Input: dimensioned drawing with shaded views. Units: mm. Origin: part minimum x, y, z. Coordinates: 2 decimals unless noted, no trailing zeros. Order: outer loops, then holes, each group sorted by start corner. A loop starts at its lowest first (then second) coordinate and runs counter-clockwise, first axis right, second up. Notation, with made-up numbers: (69.25, 20.25) -> (85.25, 20.25) arc R29 cw to (85.25, 48.25) -> close; hole circle Ø1 at (88.5, 59). An arc over 180 degrees is marked (long way). Answer in a Markdown table with one row per item. Add a question column.
1) Section query B-B on z = 90. Return the cut outline in (x, y).
2) Contact query for flat-ended pins moving along their axis: P1, Ø7.5, axis at y = 275, z = 90, coming from the -X side; P2, Ø3, axis at x = 100, y = 216.5, coming from the -Z side. Output: stop coordinate, or through.
3) Section query A-A on y = 280. Return the cut outline in (x, z), then the cut area to 3 significant figures.
4) Pull-direction query (X, two-part tool) for the marked faces 1, 2 and 3; classes: +X half, -X half, draft (parallel to the pull), parting line (faces both ways), or undercut.
5) Ray query, line 1 (Y direction, x = 18.5, z = 90); line 2 (Z direction, x = 6, y = 280). Return the intervals inside material, ascending. Write a range as from..to.
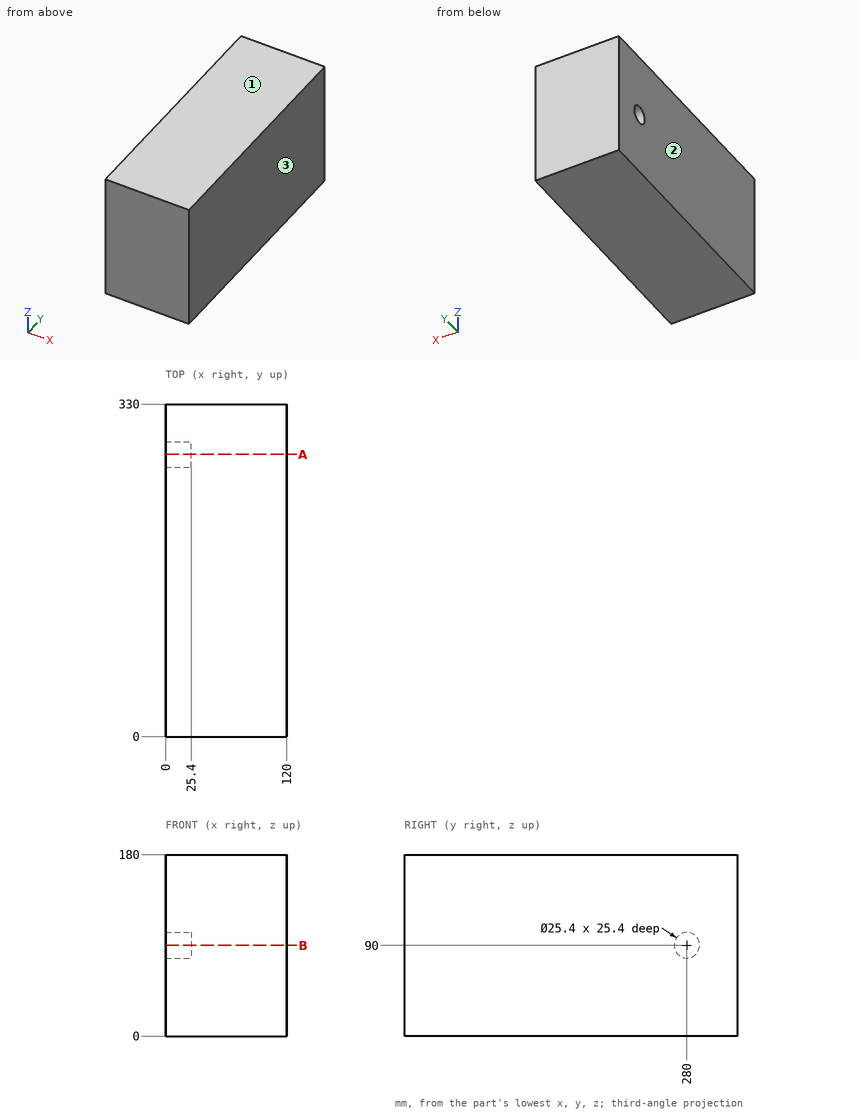
Result:
| question | item | result |
|---|---|---|
| 1 | outline | (0, 0) -> (120, 0) -> (120, 330) -> (0, 330) -> (0, 292.7) -> (25.4, 292.7) -> (25.4, 267.3) -> (0, 267.3) -> close |
| 2 | P1 | x = 25.4 |
| 2 | P2 | z = 0 |
| 3 | outline | (0, 0) -> (120, 0) -> (120, 180) -> (0, 180) -> (0, 102.7) -> (25.4, 102.7) -> (25.4, 77.3) -> (0, 77.3) -> close |
| 3 | area | 21,000 mm2 |
| 4 | face 1 | draft |
| 4 | face 2 | -X half |
| 4 | face 3 | +X half |
| 5 | line 1 | 0..267.3, 292.7..330 |
| 5 | line 2 | 0..77.3, 102.7..180 |
